from build123d import *

# Parameters (mm, degrees)
EXTRUDE_1_DEPTH     = 76
FILLET_1_R          = 38
RIB_1_REACH         = 148.127
SKETCH_4_WALL_W     = 393.877609006
SKETCH_4_WALL_H     = 5
RIB_START           = -5
RIB_2_DEPTH         = 5
SKETCH_7_R          = 2.5
CUT_EXTRUDE_1_DEPTH = 10
SKETCH_8_R          = 2.5
CUT_EXTRUDE_2_DEPTH = 10
FILLET_2_R          = 2
CHAMFER_1_SIZE      = 10
CHAMFER_1_SIZE2     = 5
FILLET_3_R          = 2
FILLET_4_R          = 2


# Read off the part's stored shape, not the designer's step: Ребро2
with BuildPart() as part:
    # Эскиз3 → Бобышка-Вытянуть1 (new body)
    with BuildSketch(Plane.XY):
        Polygon((76, 0), (0, 0), (0, 5), (71, 5), (71, 99), (76, 99), align=None)
    extrude(amount=EXTRUDE_1_DEPTH)

    # Скругление1
    fillet_1_edges = [part.edges().sort_by_distance(p)[0] for p in [
        (0, 2.5, 0),
        (0, 2.5, 76),
    ]]
    fillet(fillet_1_edges, radius=FILLET_1_R - 0.0001)  # a hair under: the kernel refuses the full size

    # Эскиз4 wall → Ребро1 (add, up to next)
    with BuildSketch(Plane(origin=(54.5, 52, 76), x_dir=(-0.331244504731, -0.94354495287, 0), z_dir=(0.94354495287, -0.331244504731, 0)), mode=Mode.PRIVATE) as rib_1_sk1:
        with Locations((0, 2.5)):
            Rectangle(SKETCH_4_WALL_W, SKETCH_4_WALL_H)
    rib_1_tool1 = extrude(rib_1_sk1.sketch, amount=RIB_1_REACH, mode=Mode.PRIVATE) - part.part
    add(rib_1_tool1.solids().sort_by_distance((54.5, 52, 76))[0])

    # Ребро2 outline → Ребро2 (add)
    with BuildSketch(Plane(origin=(0, 0, 0), x_dir=(-1, 0, 0), z_dir=(0, 0, -1)).offset(RIB_START)):
        Polygon((-38, 5), (-71, 99), (-71, 5), align=None)
    extrude(amount=RIB_2_DEPTH)

    # Эскиз7 → Вырез-Вытянуть1 (cut)
    with BuildSketch(Plane(origin=(0, 5, 0), x_dir=(1, 0, 0), z_dir=(0, 1, 0))):
        with Locations(Location((20, -38, 0), (0, 0, 180))):
            Circle(SKETCH_7_R)
        with Locations(Location((29, -22.411542732, 0), (0, 0, 180))):
            Circle(SKETCH_7_R)
        with Locations(Location((47, -22.411542732, 0), (0, 0, 180))):
            Circle(SKETCH_7_R)
        with Locations(Location((56, -38, 0), (0, 0, 180))):
            Circle(SKETCH_7_R)
        with Locations(Location((47, -53.588457268, 0), (0, 0, 180))):
            Circle(SKETCH_7_R)
        with Locations(Location((29, -53.588457268, 0), (0, 0, 180))):
            Circle(SKETCH_7_R)
    extrude(amount=-CUT_EXTRUDE_1_DEPTH, mode=Mode.SUBTRACT)

    # Эскиз8 → Вырез-Вытянуть2 (cut)
    with BuildSketch(Plane(origin=(76, 0, 0), x_dir=(0, 0, -1), z_dir=(1, 0, 0))):
        with Locations((-38, 52)):
            Circle(SKETCH_8_R)
        with Locations((-53.588457268, 61)):
            Circle(SKETCH_8_R)
        with Locations((-53.588457268, 79)):
            Circle(SKETCH_8_R)
        with Locations((-38, 88)):
            Circle(SKETCH_8_R)
        with Locations((-22.411542732, 79)):
            Circle(SKETCH_8_R)
        with Locations((-22.411542732, 61)):
            Circle(SKETCH_8_R)
    extrude(amount=-CUT_EXTRUDE_2_DEPTH, mode=Mode.SUBTRACT)

    # Скругление2
    fillet_2_edges = [part.edges().sort_by_distance(p)[0] for p in [
        (76, 0, 38),
    ]]
    fillet(fillet_2_edges, radius=FILLET_2_R)

    # Фаска1
    chamfer_1_edges = [part.edges().sort_by_distance(p)[0] for p in [
        (71, 5, 38),
    ]]
    chamfer_1_side = [part.faces().sort_by_distance(p)[0] for p in [
        (71, 52, 6.148564321),
    ]]
    chamfer(chamfer_1_edges, length=CHAMFER_1_SIZE, length2=CHAMFER_1_SIZE2, reference=chamfer_1_side[0])

    # Скругление3
    fillet_3_edges = [part.edges().sort_by_distance(p)[0] for p in [
        (38, 5, 73.5),
        (38, 5, 2.5),
    ]]
    fillet(fillet_3_edges, radius=FILLET_3_R)

    # Скругление4
    fillet_4_edges = [part.edges().sort_by_distance(p)[0] for p in [
        (73.5, 99, 76),
        (73.5, 99, 0),
    ]]
    fillet(fillet_4_edges, radius=FILLET_4_R)


solid = part.part
Geometry check sheet. Reference: the model listing, model coordinates, mm. A direction names the side the tool comes from. Round coordinates to 2 decimals unless told otherwise and drop trailing zeros. Loops run counter-clockwise (first coordinate to the right, second up) from the corner with the lowest first, then second, coordinate; pieces in that order, holes last.
Item 1: Cross-section at B-B on x = 19. Record the boundary of the cut face in (y, z), then the cut area to 3 significant figures.
Item 2: Cross-section at C-C on x = 47. Record the boundary of the cut face in (y, z), then the cut area to 3 significant figures.
Item 3: Mould release check, pull along Y, two halves, no side actions. Record for faces 1 (the cylindrical face through (73.535, 61.11, 56.086)), 2 (the flat face through (60, 39, 71)), 3 (the flat face through (54.962, 53.317, 73.465)), 4 (the flat face through (38, 0, 37)): pulls with the +Y half, pulls with the -Y half, needs draft (parallel to the pull), parting line crosses it, or undercut.
Item 4: Cross-section at A-A on y = 52. Record the boundary of the cut face in (x, z).
Item 5: Gauge pin test, flat ends, axial feed: pin 1 (20 mm diameter, centred on y = 42.5, z = 34.5, fed in from -X); pin 2 (17 mm diameter, centred on x = 49, y = 62.5, fed in from +Z); pin 3 (6 mm diameter, centred on x = 10.5, z = 57.5, fed in from +Y). Record the tip position at first contact, or that the pin passes through.
Item 6: Thickness scan on line 1 (Y direction, x = 73.65, z = 38); line 2 (Z direction, x = 46.5, y = 9); line 3 (X direction, y = 36, z = 30). Record the ranges inside material, lowest first.
Item 7: Access from +Z, -Z, +X, -X, +Y, -Y to the whole of each face (thin tool, end or side, straight path). Record for faces 5 (the cylindrical face through (22, 2.5, 36.5)), 6 (the flat face through (62, 32, 5)).
Item 8: Cross-section at D-D on z = 43. Record the boundary of the cut face in (x, y), then the cut area to 3 significant figures.
Answer sheet:
1. outline: (0, 5.09) - (5, 5.09) - (5, 35.71) - (0, 35.71) - close; (0, 40.29) - (5, 40.29) - (5, 70.91) - (0, 70.91) - close
1. area: 306 mm2
2. outline: (0, 0) - (30.64, 0) - (30.64, 5) - (5, 5) - (5, 19.91) - (0, 19.91) - close; (0, 24.91) - (5, 24.91) - (5, 51.09) - (0, 51.09) - close; (0, 56.09) - (5, 56.09) - (5, 71) - (30.64, 71) - (30.64, 76) - (0, 76) - close
2. area: 586 mm2
3. face 1: undercut
3. face 2: needs draft
3. face 3: pulls with the +Y half
3. face 4: pulls with the -Y half
4. outline: (54.5, 0) - (76, 0) - (76, 35.5) - (71, 35.5) - (71, 5) - (54.5, 5) - close; (54.5, 71) - (71, 71) - (71, 40.5) - (76, 40.5) - (76, 76) - (54.5, 76) - close
5. pin 1: stops at x = 71
5. pin 2: passes through
5. pin 3: stops at y = 5
6. line 1: y = 0 to 49.5, 54.5 to 85.5, 90.5 to 99
6. line 2: z = 0 to 5, 71 to 76
6. line 3: x = 71 to 76
7. face 5: +Y, -Y
7. face 6: -X, +Y
8. outline: (0.33, 0) - (74, 0) arc R2 ccw to (76, 2) - (76, 99) - (71, 99) - (71, 15) - (66, 5) - (0.33, 5) - close
8. area: 872 mm2
